```python
from build123d import *

# Parameters (mm, degrees)
F0_R          = 5.08
F0_R_2        = 4.064
F1_DEPTH      = 12.7
F2_W          = 1.524
F2_H          = 2.54
F3_DEPTH      = 25.4
F5_END_RADIUS = 5.08
F4_W          = 2.286
F4_H          = 1.905
F5_REACH      = 8.0567051265
F6_END_RADIUS = 4.064
F6_REACH      = 8.0567051265


with BuildPart() as f1:
    # F0 (on Top) → F1 (new body)
    with BuildSketch(Plane.XY):
        Circle(F0_R)
        Circle(F0_R_2, mode=Mode.SUBTRACT)
    extrude(amount=F1_DEPTH)

    # F2 (on Front) → F3 (cut)
    with BuildSketch(Plane.XZ):
        with Locations((0, 11.43)):
            Rectangle(F2_W, F2_H)
    extrude(amount=F3_DEPTH, mode=Mode.SUBTRACT)

    f5_end = (Plane(origin=(0, 0, 6.35), x_dir=(-1, 0, 0), z_dir=(0, 0, -1)) * Cylinder(F5_END_RADIUS, 54.4665691842, mode=Mode.PRIVATE)).faces().sort_by_distance((-5.08, 0, 6.35))[0]
    # F4 (on Front) → F5 (join, up to the whole of a round face its end follows)
    with BuildSketch(Plane.XZ):
        with Locations((0, -0.9525)):
            Rectangle(F4_W, F4_H)
    f5_long = extrude(amount=F5_REACH, mode=Mode.PRIVATE)
    add(split(f5_long, bisect_by=f5_end, keep=Keep.BOTTOM, mode=Mode.PRIVATE))

    f6_end = (Plane(origin=(0, 0, 6.35), x_dir=(-1, 0, 0), z_dir=(0, 0, -1)) * Cylinder(F6_END_RADIUS, 57.0893653975, mode=Mode.PRIVATE)).faces().sort_by_distance((-4.064, 0, 6.35))[0]
    # F4 (on Front) → F6 (cut, up to the whole of a round face its end follows)
    with BuildSketch(Plane.XZ):
        with Locations((0, -0.9525)):
            Rectangle(F4_W, F4_H)
    f6_long = extrude(amount=F6_REACH, mode=Mode.PRIVATE)
    add(split(f6_long, bisect_by=f6_end, keep=Keep.BOTTOM, mode=Mode.PRIVATE), mode=Mode.SUBTRACT)


solid = f1.part
```
Verification items for the finished model (mm, model axes). A direction names the side the tool comes from. Coordinates: 2 decimals unless noted, no trailing zeros. Loops run counter-clockwise (first coordinate to the right, second up) from the corner with the lowest first, then second, coordinate; pieces in that order, holes last. Notation, with made-up numbers: (33, -39) -> (68, -39) arc R16 cw to (68, -12) -> close; hole circle Ø11 at (37, -10). An arc over 180 degrees is marked (long way). Answer in a Markdown table with one row per item. Add a question column.
1. Section check C-C, the plane z = 4.75. Enter the section's corners in (x, y), then the cut area to 3 significant figures.
2. Section check B-B, the plane x = -2.25. Enter the section's corners in (y, z).
3. Depth check by flat-ended pin: P1, Ø2, axis at x = -3, z = 9, coming from the +Y side; P2, Ø2, axis at y = -2, z = 0, coming from the -X side; P3, Ø0.5, axis at y = -4.5, z = 11.5, coming from the -X side. Enter the tip coordinate at first touch or a pass-through.
4. Access from +Z, -Z, +X, -X, +Y, -Y to the whole of each face (thin tool, end or side, straight path). Record for faces 3 (the face through (0.762, -4.5, 11.4)), 4 (the face through (-1.143, -4.4, -1)), 5 (the face through (1.143, -4.4, -1)).
5. Section check D-D, the plane y = 4.5. Enter the section's corners in (x, z).
6. Section check A-A, the plane y = 0. Enter the section's corners in (x, z).
7. Material ranges on probe 1 along X at (y, z) = (0, 9); probe 2 along Z at (x, y) = (-2.25, 4), recorded low to high. Write a range as [from, to].
8. Draft check along Y on faces 1 (the face through (1.875, 3.605, 5.295)), 2 (the face through (-2, 4, 0)). Enter one of: +Y half, -Y half, draft (parallel to the pull), parting line (faces both ways), or undercut.
Derived:
| question | item | result |
|---|---|---|
| 1 | outline | circle Ø10.16 at (0, 0); hole circle Ø8.13 at (0, 0) |
| 1 | area | 29.2 mm² |
| 2 | outline | (-4.55, 0) -> (-3.38, 0) -> (-3.38, 12.7) -> (-4.55, 12.7) -> close; (3.38, 0) -> (4.55, 0) -> (4.55, 12.7) -> (3.38, 12.7) -> close |
| 3 | P1 | stops at y = 4.67 |
| 3 | P2 | stops at x = -4.98 |
| 3 | P3 | stops at x = -2.78 |
| 4 | face 3 | +Z, -Y |
| 4 | face 4 | -Z, -X, +Y, -Y |
| 4 | face 5 | -Z, +X, +Y, -Y |
| 5 | outline | (-2.36, 0) -> (2.36, 0) -> (2.36, 12.7) -> (-2.36, 12.7) -> close |
| 6 | outline | (-5.08, 0) -> (-4.06, 0) -> (-4.06, 12.7) -> (-5.08, 12.7) -> close; (4.06, 0) -> (5.08, 0) -> (5.08, 12.7) -> (4.06, 12.7) -> close |
| 7 | probe 1 | x = [-5.08, -4.06], [4.06, 5.08] |
| 7 | probe 2 | z = [0, 12.7] |
| 8 | face 1 | undercut |
| 8 | face 2 | draft |
